Verification items for the finished model (mm, model axes). Face numbers are marked on the shaded views. A direction names the side the tool comes from. Round coordinates to 2 decimals unless told otherwise and drop trailing zeros. Order: outer loops, then holes, each group sorted by start corner. A loop starts at its lowest first (then second) coordinate and runs counter-clockwise, first axis right, second up. Notation, with made-up numbers: (67, -0.5) -> (84, -0.5) arc R11 ccw to (84, 5.5) -> close; hole circle Ø7 at (3, 14). An arc over 180 degrees is marked (long way). Return JSON: item names as keys, results as strings. Group by question number.
1) Draft check along Y on the marked faces 1, 2, 3 and 4. Enter one of: pulls with the +Y half, pulls with the -Y half, needs draft (parallel to the pull), parting line crosses it, or undercut.
2) Scan lines: L1, parallel to X at y = 235, z = 53.5; L2, parallel to Z at x = -370.5, y = 144.5. Record each from-to range of solid material in increasing order.
3) Section check C-C on z = 63. State how many separate pieces and enclosed holes the cut face has, plus the area to 3 significant figures.
4) Section check A-A on y = -268.5. Enter the section's corners in (x, z), plus the area to 3 significant figures.
5) Tool access check on the marked faces 5 and 6. Record the directions out of +Z, -Z, +X, -X, +Y, -Y that give a thin tool (end or side, any length) a straight path to the whole face; none if there is none.
```python
from build123d import *

# Parameters (mm, degrees)
F0_W     = 1000
F0_H     = 1000
F1_DEPTH = 100
F2_W     = 300
F2_H     = 300
F3_DEPTH = 50


with BuildPart() as f1:
    # F0 (on Top) → F1 (new body)
    with BuildSketch(Plane.XY):
        Rectangle(F0_W, F0_H)
    extrude(amount=F1_DEPTH)

    # F2 (on face) → F3 (cut)
    with BuildSketch(Plane.XY.offset(100)):
        with Locations((-325, 325)):
            Rectangle(F2_W, F2_H)
        with Locations((0, 325)):
            Rectangle(F2_W, F2_H)
        with Locations((325, 325)):
            Rectangle(F2_W, F2_H)
        with Locations((325, 0)):
            Rectangle(F2_W, F2_H)
        Rectangle(F2_W, F2_H)
        with Locations((-325, 0)):
            Rectangle(F2_W, F2_H)
        with Locations((-325, -325)):
            Rectangle(F2_W, F2_H)
        with Locations((0, -325)):
            Rectangle(F2_W, F2_H)
        with Locations((325, -325)):
            Rectangle(F2_W, F2_H)
    extrude(amount=-F3_DEPTH, mode=Mode.SUBTRACT)


solid = f1.part
```
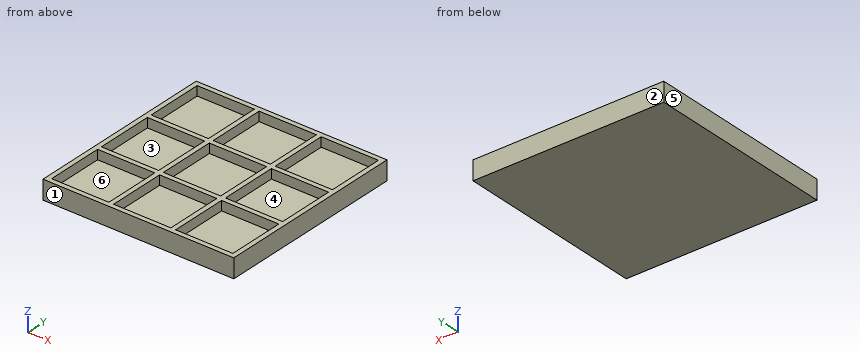
Check result:
{
 "1": {"face 1": "pulls with the -Y half", "face 2": "pulls with the +Y half", "face 3": "undercut", "face 4": "undercut"},
 "2": {"L1": "-500 to -475, -175 to -150, 150 to 175, 475 to 500", "L2": "0 to 50"},
 "3": {"separate pieces": "1", "enclosed holes": "9", "area": "190,000 mm^2"},
 "4": {"outline": "(-500, 0) -> (500, 0) -> (500, 100) -> (475, 100) -> (475, 50) -> (175, 50) -> (175, 100) -> (150, 100) -> (150, 50) -> (-150, 50) -> (-150, 100) -> (-175, 100) -> (-175, 50) -> (-475, 50) -> (-475, 100) -> (-500, 100) -> close", "area": "55,000 mm^2"},
 "5": {"face 5": "+Z, -Z, -X, +Y, -Y", "face 6": "+Z"}
}
